Here's how the part is built. I have some questions about the finished solid (model axes, mm). Face numbers are marked on the shaded views. A direction names the side the tool comes from. Coordinates: 2 decimals unless noted, no trailing zeros. Write each loop counter-clockwise with the first axis right and the second up, starting at its lowest first coordinate (ties: lowest second). Pieces come first, ordered by that corner, then holes.
(1) Imagine slicing it at C-C, the plane x = -55. List the corners of the cut face in (y, z) for me.
(2) Imagine slicing it at B-B, the plane z = -18. List the corners of the cut face in (x, y) for me, plus the area to 3 significant figures.
(3) Imagine slicing it at A-A, the plane y = -9. List the corners of the cut face in (x, z) for me.
(4) Please list where these lines run through material, in increasing order: probe 1 along X at (y, z) = (-86.5, -15.5); probe 2 along X at (y, z) = (-19.5, 172.5); probe 3 along Z at (x, y) = (105.5, -44.5).
(5) Which directions (+Z, -Z, +X, -X, +Y, -Y) give clear straight access to the entire face, cutting with the end or side of a thin tool? Please do the marked faces 1 and 2.
(6) For pin 1 Ø5 at (x, y) = (122, -43) entering from +Z; pin 2 Ø5 at (y, z) = (-74.5, 127.5) entering from +X; pin 3 Ø22.5 at (y, z) = (-53, -53.5) entering from +X, each with a flat end and sliding along its axis, tell me the tip position at first contact or that it passes through.
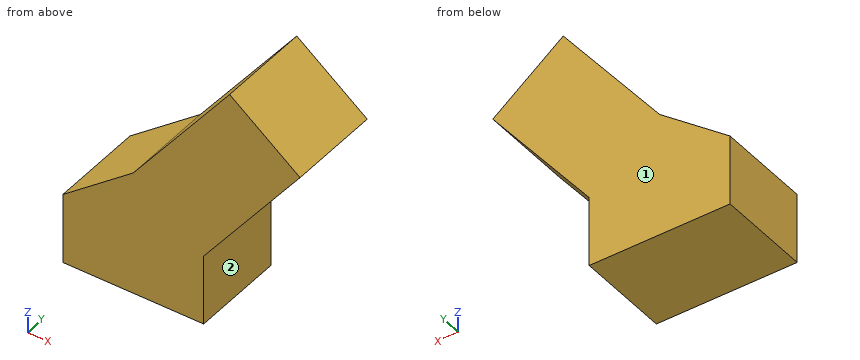
```python
from build123d import *

# Parameters (mm, degrees)
F0_W     = 148.616835475
F0_H     = 74.3084251881
F1_DEPTH = 100
F2_DEPTH = 166.5562391281


with BuildPart() as f1:
    # F0 (on Front) → F1 (new body)
    with BuildSketch(Plane.XZ):
        Polygon((0, 57.283565402), (-74.3084102869, 0), (74.3084251881, 0), align=None)
        with Locations((7.4506e-06, -37.154212594)):
            Rectangle(F0_W, F0_H)
    extrude(amount=F1_DEPTH)

    # F2 (add): a face of the model
    f2_faces = [f1.faces().sort_by_distance(p)[0] for p in [
        (37.154212594, -50, 28.641782701),
    ]]
    extrude(f2_faces, amount=F2_DEPTH)


solid = f1.part
```
Recorded:
1. outline: (-100, -74.31) - (0, -74.31) - (0, 14.88) - (-100, 14.88) - close
2. outline: (-74.31, -100) - (74.31, -100) - (74.31, 0) - (-74.31, 0) - close
2. area: 14,900 mm2
3. outline: (-74.31, -74.31) - (74.31, -74.31) - (74.31, 0) - (176, 131.91) - (101.69, 189.19) - (0, 57.28) - (-74.31, 0) - close
4. probe 1: x = -74.31 to 74.31
4. probe 2: x = 88.82 to 123.34
4. probe 3: z = 40.46 to 186.26
5. face 1: +Z, -Z, +X, -X, +Y
5. face 2: -Z, +X, +Y, -Y
6. pin 1: stops at z = 175.46
6. pin 2: stops at x = 174.52
6. pin 3: stops at x = 74.31
